Check sheet for the drawn part. Datum: minimum x, y, z corner. Units: mm. Give positions to 0.01 mm unless a question says otherwise; leave off trailing zeros. Write each loop counter-clockwise with the first axis right and the second up, starting at its lowest first coordinate (ties: lowest second). Pieces come first, ordered by that corner, then holes. Notation, with made-up numbers: M 88.5,73.25 L 118.5,73.25 A25 cw 118.5,107.25 Z; hole C -37.5,-25 d1. An arc over 180 degrees is marked long. Write item = value, one per line.
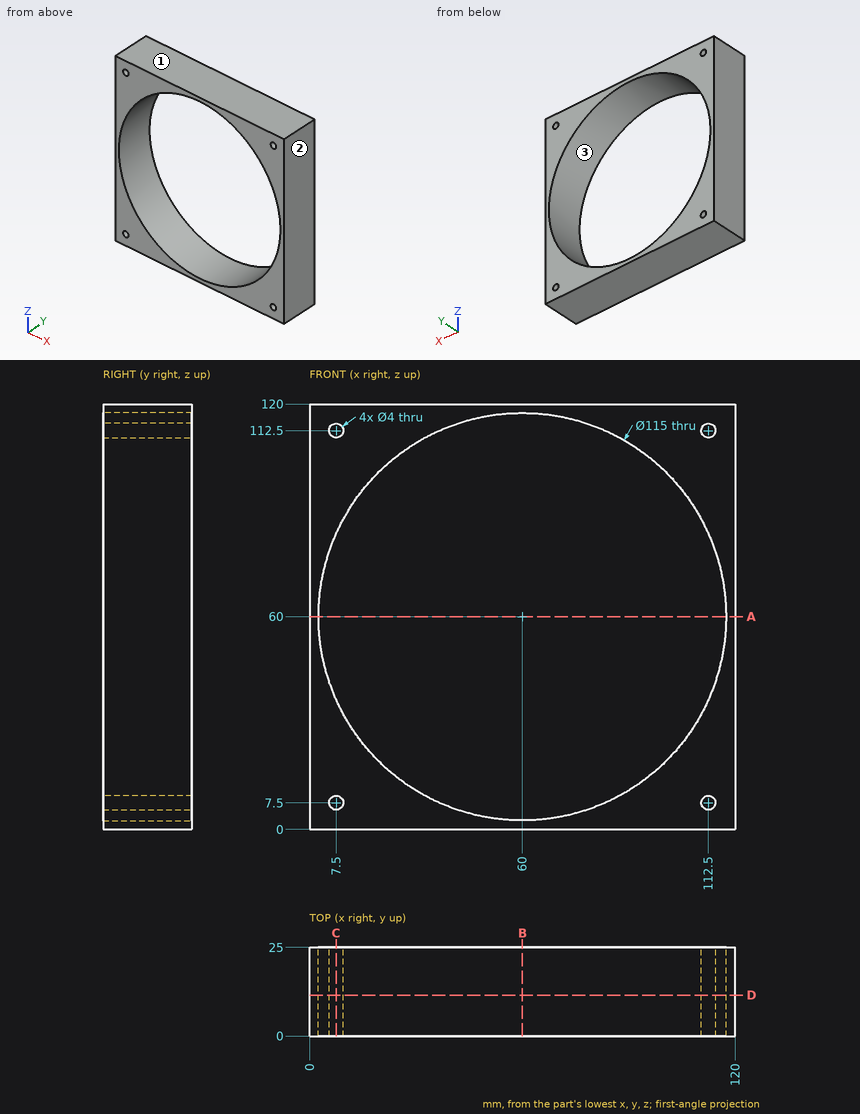
1) Cross-section at C-C on x = 7.5. Record the boundary of the cut face in (y, z), plus the area to 3 significant figures.
From the geometry:
outline = M 0,0 L 25,0 L 25,5.5 L 0,5.5 Z; M 0,9.5 L 25,9.5 L 25,36.55 L 0,36.55 Z; M 0,83.45 L 25,83.45 L 25,110.5 L 0,110.5 Z; M 0,114.5 L 25,114.5 L 25,120 L 0,120 Z
area = 1,630 mm^2
2) Cross-section at A-A on z = 60. Record the boundary of the cut face in (x, y), plus the area to 3 significant figures.
From the geometry:
outline = M 0,0 L 2.5,0 L 2.5,25 L 0,25 Z; M 117.5,0 L 120,0 L 120,25 L 117.5,25 Z
area = 125 mm^2
3) Cross-section at D-D on y = 11.5. Record the boundary of the cut face in (x, z), plus the area to 3 significant figures.
From the geometry:
outline = M 0,0 L 120,0 L 120,120 L 0,120 Z; hole C 60,60 d115; hole C 7.5,7.5 d4; hole C 7.5,112.5 d4; hole C 112.5,7.5 d4; hole C 112.5,112.5 d4
area = 3,960 mm^2
4) Draft check along Z on the marked faces 1, 2 and 3. Enter one of: +Z half, -Z half, draft (parallel to the pull), parting line (faces both ways), or undercut.
From the geometry:
face_1 = +Z half
face_2 = draft
face_3 = undercut
5) Cross-section at B-B on x = 60. Record the boundary of the cut face in (y, z), plus the area to 3 significant figures.
From the geometry:
outline = M 0,0 L 25,0 L 25,2.5 L 0,2.5 Z; M 0,117.5 L 25,117.5 L 25,120 L 0,120 Z
area = 125 mm^2
6) Material ranges on probe 1 along X at (y, z) = (8.25, 60); probe 2 along X at (y, z) = (14.75, 112.5); probe 3 along Z at (x, y) = (113, 7.5), recorded low to high. Write a range as from..to.
From the geometry:
probe_1 = 0..2.5, 117.5..120
probe_2 = 0..5.5, 9.5..36.55, 83.45..110.5, 114.5..120
probe_3 = 0..5.56, 9.44..37.7, 82.3..110.56, 114.44..120
